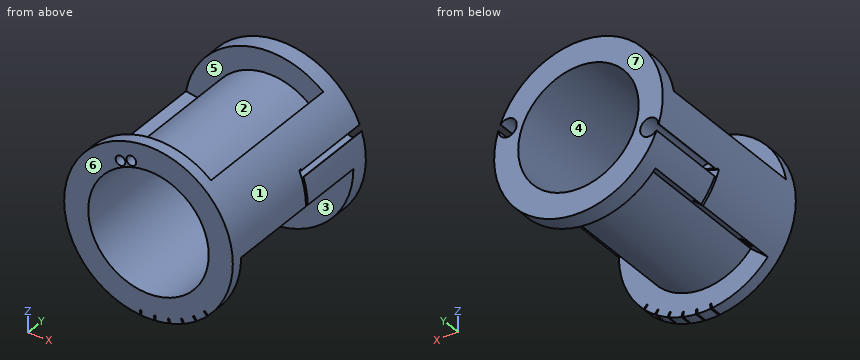
```python
from build123d import *

# Parameters (mm, degrees)
SKETCH1_W                    = 25.4
SKETCH1_H                    = 203.2
SKETCH2_W                    = 23.400004
SKETCH2_H                    = 171.45
CUT_REVOLVE1_ANGLE           = 140
SKETCH5_R                    = 9.525
CUT_EXTRUDE1_DEPTH           = 88.9
SKETCH7_W                    = 12.7
SKETCH7_H                    = 2.54
CUT_REVOLVE3_ANGLE           = 23
FILLET2_R                    = 0.254
FILLET2_OF_MIRROR1_R         = 0.254
CUT_EXTRUDE6_DEPTH           = 12.7
CIRPATTERN1_COUNT            = 6
CIRPATTERN1_ANGLE            = 50
SKETCH12_R                   = 5.08
CUT_EXTRUDE7_DEPTH           = 12.7
SKETCH16_W                   = 23.368
SKETCH16_H                   = 171.45
CUT_REVOLVE4_ANGLE           = 60
CUT_REVOLVE4_OTHER_WAY_ANGLE = 60
SKETCH17_R                   = 6.35


with BuildPart() as part:
    # Sketch1 → Revolve1 (revolve)
    with BuildSketch(Plane.XY):
        with Locations((76.2, 101.6)):
            Rectangle(SKETCH1_W, SKETCH1_H)
    revolve(axis=Axis((0, 0, 0), (0, 1, 0)))

    # Sketch2 → Cut-Revolve1 (revolve, cut)
    with BuildSketch(Plane.XY):
        with Locations((77.199998, 98.425)):
            Rectangle(SKETCH2_W, SKETCH2_H)
    revolve(axis=Axis((0, 0, 0), (0, 1, 0)), revolution_arc=CUT_REVOLVE1_ANGLE, mode=Mode.SUBTRACT)

    # Sketch5 → Cut-Extrude1 (cut)
    with BuildSketch(Plane(origin=(0, 203.2, 0), x_dir=(1, 0, 0), z_dir=(0, 1, 0))):
        with Locations((-74.600035871, 27.152192532)):
            Circle(SKETCH5_R)
    cut_extrude1 = extrude(amount=-CUT_EXTRUDE1_DEPTH, mode=Mode.SUBTRACT)

    # Sketch7 → Cut-Revolve3 (revolve, cut)
    with BuildSketch(Plane(origin=(0, 0, 0), x_dir=(-0.766044443, 0, -0.64278761), z_dir=(0.64278761, 0, -0.766044443))):
        with Locations((82.55, 113.03)):
            Rectangle(SKETCH7_W, SKETCH7_H)
    cut_revolve3 = revolve(axis=Axis((0, 213.36, 0), (0, 1, 0)), revolution_arc=CUT_REVOLVE3_ANGLE, mode=Mode.SUBTRACT)

    # Fillet2
    fillet2_edges = [part.edges().sort_by_distance(p)[0] for p in [
        (-83.359280525, 158.75, -30.894018036),
        (-83.715205635, 158.75, -29.916121832),
    ]]
    fillet(fillet2_edges, radius=FILLET2_R)

    # Mirror1: Cut-Extrude1, Cut-Revolve3 across plane
    add(cut_extrude1.mirror(Plane(origin=(0, 0, 0), x_dir=(-0.342020143, 0, 0.939692621), z_dir=(-0.939692621, 0, -0.342020143))), mode=Mode.SUBTRACT)
    add(cut_revolve3.mirror(Plane(origin=(0, 0, 0), x_dir=(-0.342020143, 0, 0.939692621), z_dir=(-0.939692621, 0, -0.342020143))), mode=Mode.SUBTRACT)

    # Fillet2 of Mirror1
    fillet2_of_mirror1_edges = [part.edges().sort_by_distance(p)[0] for p in [
        (83.715205635, 158.75, 29.916121832),
        (83.359280525, 158.75, 30.894018036),
    ]]
    fillet(fillet2_of_mirror1_edges, radius=FILLET2_OF_MIRROR1_R)

    # Sketch15 → Cut-Extrude6 (cut)
    with BuildSketch(Plane(origin=(0, 12.7, 0), x_dir=(1, 0, 0), z_dir=(0, 1, 0))):
        with BuildLine():
            Line((59.269690399, 59.269690399), (62.861792847, 62.861792847))
            ThreePointArc((62.861792847, 62.861792847), (62.310833596, 63.40796493), (61.755129134, 63.94930825))
            Line((61.755129134, 63.94930825), (58.226264612, 60.295062064))
            ThreePointArc((58.226264612, 60.295062064), (58.750214534, 59.784652648), (59.269690399, 59.269690399))
        make_face()
    cut_extrude6 = extrude(amount=-CUT_EXTRUDE6_DEPTH, mode=Mode.SUBTRACT)

    # CirPattern1: Cut-Extrude6 ×6 about axis
    cirpattern1_axis = Axis((0, 0, 0), (0, 1, 0))
    for i in range(1, CIRPATTERN1_COUNT):
        add(cut_extrude6.rotate(cirpattern1_axis, i * CIRPATTERN1_ANGLE / (CIRPATTERN1_COUNT - 1)), mode=Mode.SUBTRACT)

    # Sketch12 → Cut-Extrude7 (cut)
    with BuildSketch(Plane(origin=(0, 12.7, 0), x_dir=(1, 0, 0), z_dir=(0, 1, 0))):
        with Locations((-29.519885583, -63.305598925)):
            Circle(SKETCH12_R)
        with Locations((-18.0785103, -67.469918966)):
            Circle(SKETCH12_R)
    extrude(amount=-CUT_EXTRUDE7_DEPTH, mode=Mode.SUBTRACT)

    # Sketch16 → Cut-Revolve4 (revolve, cut)
    with BuildSketch(Plane(origin=(0, 0, 0), x_dir=(-0.342020143, 0, 0.939692621), z_dir=(-0.939692621, 0, -0.342020143))):
        with Locations((77.216, 98.425)):
            Rectangle(SKETCH16_W, SKETCH16_H)
    revolve(axis=Axis((0, -7.62, 0), (0, 1, 0)), revolution_arc=CUT_REVOLVE4_ANGLE, mode=Mode.SUBTRACT)

    # Sketch16 → Cut-Revolve4 other way (revolve, cut)
    with BuildSketch(Plane(origin=(0, 0, 0), x_dir=(-0.342020143, 0, 0.939692621), z_dir=(-0.939692621, 0, -0.342020143))):
        with Locations((77.216, 98.425)):
            Rectangle(SKETCH16_W, SKETCH16_H)
    revolve(axis=Axis((0, -7.62, 0), (0, -1, 0)), revolution_arc=CUT_REVOLVE4_OTHER_WAY_ANGLE, mode=Mode.SUBTRACT)

    # Sketch17 → Cut-Revolve5 (revolve, cut)
    with BuildSketch(Plane(origin=(0, 0, 0), x_dir=(-0.342020143, 0, 0.939692621), z_dir=(-0.939692621, 0, -0.342020143))):
        with Locations((76.2, 31.75)):
            Circle(SKETCH17_R)
    revolve(axis=Axis((0, 213.36, 0), (0, -1, 0)), mode=Mode.SUBTRACT)


solid = part.part
```
Here's how the part is built. I have some questions about the finished solid (model axes, mm). Face numbers are marked on the shaded views. A direction names the side the tool comes from. Coordinates: 2 decimals unless noted, no trailing zeros. Order: outer loops, then holes, each group sorted by start corner. A loop starts at its lowest first (then second) coordinate and runs counter-clockwise, first axis right, second up.
Item 1: If we section it at A-A, the plane x = 0: List the corners of the cut face in (y, z) for me.
Response values:
outline: (0, -88.9) - (12.7, -88.9) - (12.7, -65.5) - (184.15, -65.5) - (184.15, -88.9) - (203.2, -88.9) - (203.2, -63.5) - (0, -63.5) - close; (0, 63.5) - (203.2, 63.5) - (203.2, 88.9) - (184.15, 88.9) - (184.15, 65.53) - (12.7, 65.53) - (12.7, 88.9) - (0, 88.9) - close
Item 2: If we section it at B-B, the plane y = 53.5: List the corners of the cut face in (x, z) for me.
Response values:
outline: (-87.55, 15.44) arc R88.9 ccw to (-68.1, -57.14) - (-50.18, -42.1) arc R65.5 ccw to (65.5, 0) - (88.9, 0) arc R88.9 ccw to (57.14, 68.1) - (42.12, 50.2) arc R65.53 ccw to (-64.54, 11.38) - close; hole circle Ø127 at (0, 0)
Item 3: I'm going to push flat-ended pins straight in: pin 1 Ø4 at (x, y) = (-20, 98) entering from -Z; pin 2 Ø8.5 at (x, z) = (-77, -25) entering from +Y; pin 3 Ø8 at (x, z) = (-18.08, 67.47) entering from -Y. Where does each tip first touch, or does it pass through?
Response values:
pin 1: stops at z = -62.98
pin 2: stops at y = 114.3
pin 3: stops at y = 184.15
Item 4: I need wall thicknesses on probe 1 along Y at (x, z) = (67, -24); probe 2 along Z at (x, y) = (0, 71); probe 3 along X at (y, z) = (192.5, 1). Which ranges of each line are inside material? Lowest first, please.
Response values:
probe 1: y = 0 to 12.7, 184.15 to 203.2
probe 2: z = -65.5 to -63.5, 63.5 to 65.53
probe 3: x = -88.89 to -63.49, 63.49 to 88.89
Item 5: Which directions (+Z, -Z, +X, -X, +Y, -Y) give clear straight access to the entire face, cutting with the end or side of a thin tool? Please do the marked faces 1, 2 and 3.
Response values:
face 1: +Y, -Y
face 2: +Z
face 3: -Z
Item 6: Thinking about a two-plate mould opening in Y: for the marked faces 4, 5, 6 and 7, which applies, pulls with the +Y half, pulls with the -Y half, needs draft (parallel to the pull), parting line crosses it, or undercut?
Response values:
face 4: needs draft
face 5: undercut
face 6: pulls with the -Y half
face 7: pulls with the +Y half
